Geometry: see drawing. Coordinates: mm, zero at the bounding-box minimum. A direction names the side the tool comes from. Give positions to 0.01 mm unless a question says otherwise; leave off trailing zeros. Loops run counter-clockwise (first coordinate to the right, second up) from the corner with the lowest first, then second, coordinate; pieces in that order, holes last. Notation, with made-up numbers: (-24, -39) - (-8, -39) arc R28 cw to (-8, -21) - close; hole circle Ø4 at (-8.75, 84.5). An arc over 180 degrees is marked (long way). Use CSV: the item, a comma, the result in double quotes. Start each with the question number.
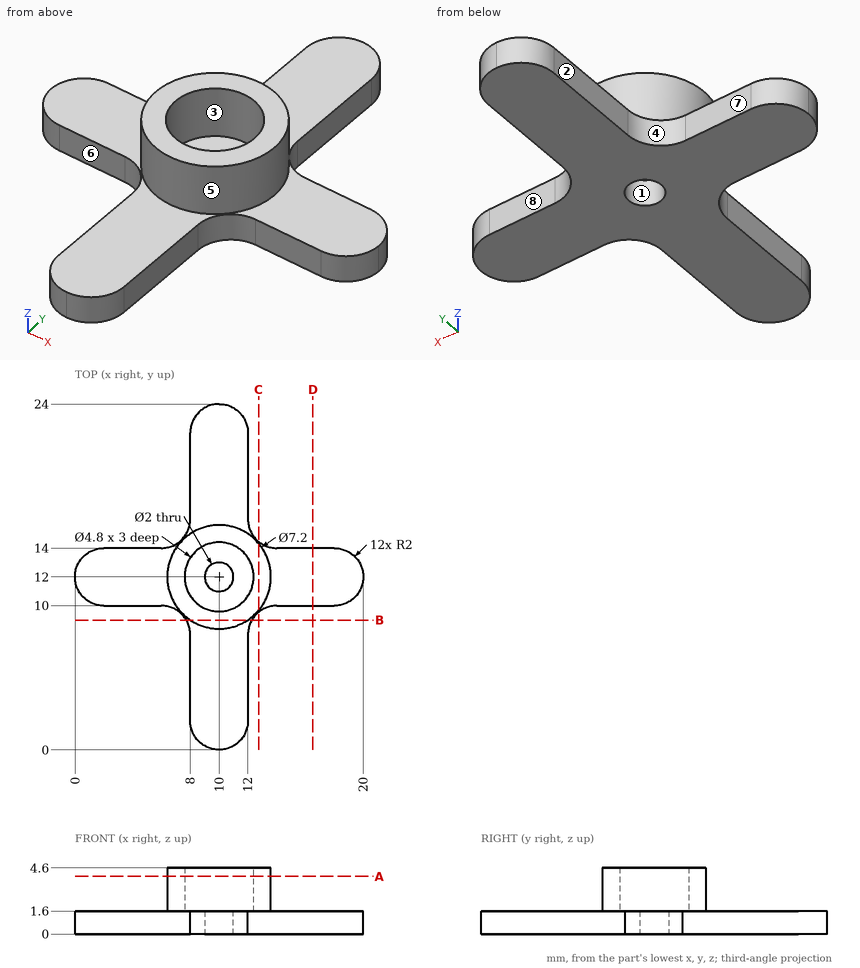
Item 1: Section A-A (z = 4). Output: boundary loops of the cut face in (x, y).
Item 2: Section B-B (y = 9). Output: boundary loops of the cut face in (x, z), plus the area to 3 significant figures.
Item 3: Section D-D (x = 16.5). Output: boundary loops of the cut face in (y, z).
Item 4: Reachability of the marked faces 5, 6, 7 and 8 from +Z, -Z, +X, -X, +Y, -Y: full face, straight path, thin tool, end or side. Return the list, or none.
Item 5: Ray query, probe 1 along Y at (x, z) = (10, 3.4); probe 2 along Y at (x, z) = (10, 0.75); probe 3 along X at (y, z) = (2.5, 0.8). Return the intervals inside material, ascending.
Item 6: Pin query (flat end, axial travel): pin 1 Ø1.8 at (x, z) = (4.5, 0.5) entering from +Y; pin 2 Ø1 at (y, z) = (13.5, 0.5) entering from -X; pin 3 Ø0.5 at (y, z) = (20.5, 0.5) entering from +X. Return the tip coordinate at first contact, or that it passes through.
Item 7: Mould query, pull axis Y, two halves, no side actions, for the marked faces 1, 2, 3 and 4. Classes: pulls with the +Y half, pulls with the -Y half, needs draft (parallel to the pull), parting line crosses it, or undercut.
Item 8: Section C-C (x = 12.75). Output: boundary loops of the cut face in (y, z).
Outcome:
1,outline,"circle Ø7.2 at (10, 12); hole circle Ø4.8 at (10, 12)"
2,outline,"(7.73, 0) - (12.27, 0) - (12.27, 1.6) - (11.99, 1.6) - (11.99, 4.6) - (8.01, 4.6) - (8.01, 1.6) - (7.73, 1.6) - close"
2,area,"19.2 mm2"
3,outline,"(10, 0) - (14, 0) - (14, 1.6) - (10, 1.6) - close"
4,face 5,"+Z"
4,face 6,"+Z, -Z, -X, -Y"
4,face 7,"+Z, -Z, -X, +Y"
4,face 8,"+Z, -Z, +X, +Y"
5,probe 1,"y = 8.4 to 9.6, 14.4 to 15.6"
5,probe 2,"y = 0 to 11, 13 to 24"
5,probe 3,"x = 8 to 12"
6,pin 1,"stops at y = 14"
6,pin 2,"stops at x = 0.27"
6,pin 3,"stops at x = 12"
7,face 1,"undercut"
7,face 2,"needs draft"
7,face 3,"undercut"
7,face 4,"pulls with the +Y half"
8,outline,"(9.56, 0) - (14.44, 0) - (14.44, 1.6) - (14.32, 1.6) - (14.32, 4.6) - (9.68, 4.6) - (9.68, 1.6) - (9.56, 1.6) - close"
